Verification items for the finished model (mm, model axes). Face numbers are marked on the shaded views. A direction names the side the tool comes from. Coordinates: 2 decimals unless noted, no trailing zeros. Write each loop counter-clockwise with the first axis right and the second up, starting at its lowest first coordinate (ties: lowest second). Pieces come first, ordered by that corner, then holes. Notation, with made-up numbers: (30.25, -26.75) -> (57.25, -26.75) arc R20 ccw to (57.25, -19.75) -> close; hole circle Ø9 at (88.25, 55.25). An arc over 180 degrees is marked (long way). Answer in a Markdown table with one row per item.
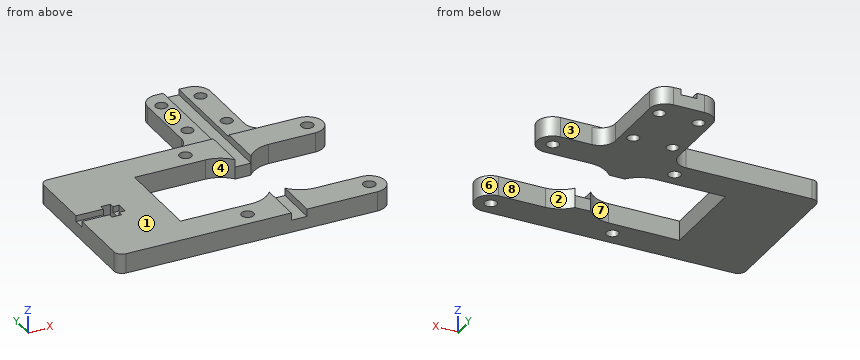
Autodesk Inventor part; units mm, degrees
ref_plane "Arbeitsebene1" through (0, 0, 5) normal (0, 0, 1) x (1, 0, 0)
ref_plane "YZ Plane" through (0, 0, 0) normal (1, 0, 0) x (0, 1, 0)
ref_plane "XZ Plane" through (0, 0, 0) normal (0, 1, 0) x (-1, 0, 0)
sketch "Skizze1" plane through (0, 0, 0) normal (0, 0, 1) x (1, 0, 0)
  line L0 (0, -27.3) -> (0, 27.3)
  line L1 (-71.7, 0) -> (34.7, 0)
  circle A0 centre (-15.5, 15.5) radius 1.55
  circle A1 centre (15.5, 15.5) radius 1.55
  circle A2 centre (-15.5, -15.5) radius 1.55
  circle A3 centre (15.5, -15.5) radius 1.55
  circle A4 centre (-16.5, 0) radius 11
  circle A5 centre (0, 0) radius 5.5
  circle A6 centre (-16.5, 0) radius 4
  arc A7 (-16.5, -7.5) -> (-16.5, 7.5) centre (-16.5, 0) ccw
  line L2 (-16.5, 7.5) -> (-36.5, 7.5)
  line L3 (-36.5, 7.5) -> (-56.5, 7.5)
  line L4 (-56.5, 7.5) -> (-56.5, -7.5)
  line L5 (-56.5, -7.5) -> (-16.5, -7.5)
  circle A8 centre (15.5, 15.5) radius 4
  circle A9 centre (-15.5, 15.5) radius 4
  line L6 (15.5, 11.5) -> (-15.5, 11.5)
  line L7 (15.5, 19.5) -> (-15.5, 19.5)
  line L8 (-15.5, 19.5) -> (-50.5, 19.5)
  line L9 (-15.5, 11.5) -> (-30.5, 11.5)
  line L10 (-50.5, 19.5) -> (-50.5, 0)
  line L11 (-30.5, 11.5) -> (-30.5, 0)
  line L12 (-15.5, -19.5) -> (-50.5, -19.5)
  line L13 (-15.5, -11.5) -> (-30.5, -11.5)
  line L14 (-50.5, -19.5) -> (-50.5, 0)
  line L15 (-30.5, -11.5) -> (-30.5, 0)
  line L16 (15.5, -11.5) -> (-15.5, -11.5)
  line L17 (15.5, -19.5) -> (-15.5, -19.5)
  line L18 (-15.5, -11.5) -> (15.5, -11.5)
  line L19 (15.5, -19.5) -> (-15.5, -19.5)
  line L20 (-30.5, -11.5) -> (15.5, -11.5)
  line L21 (15.5, -19.5) -> (-50.5, -19.5)
  arc A10 (15.5, -19.5) -> (15.5, -11.5) centre (15.5, -15.5) ccw
  point P0 (-50.5, 7.5)
  point P1 (-30.5, 7.5)
  dimension "d0" = 3.1
  dimension "d1" = 15.5
  dimension "d2" = 15.5
  dimension "d3" = 22
  dimension "d4" = 16.5
  dimension "d5" = 11
  dimension "d6" = 8
  dimension "d7" = 15
  dimension "d10" = 15
  dimension "d11" = 40
  dimension "d17" = 8
  dimension "d19" = 8
  dimension "d22" = 35
  dimension "d23" = 15
ref_plane "Arbeitsebene1" through (0, 0, 5) normal (0, 0, 1) x (1, 0, 0)
extrude "Extrusion5" add sketch "Skizze1" along normal blind 5 contours L17 L12 L14 L5 L15 L13 L16 L0 | L0 L16 A10 L17 | L14 L1 L15 L5 | L10 L3 L2 L11 L1 | L6 A9 L7 L0 | L0 L7 A8 L6 | L2 L3 L10 L8 A9 L9 L11 | A8 | A9
sketch "Skizze4" plane through (0, 0, 5) normal (0, 0, 1) x (1, 0, 0)
  line L0 (-30.5, 11.5) -> (15.5, 11.5)
  arc A0 (15.5, 11.5) -> (15.5, 19.5) centre (15.5, 15.5) ccw
  line L1 (15.5, 19.5) -> (-50.5, 19.5)
  line L2 (-50.5, 19.5) -> (-50.5, -19.5)
  line L3 (-50.5, -19.5) -> (15.5, -19.5)
  arc A1 (15.5, -19.5) -> (15.5, -11.5) centre (15.5, -15.5) ccw
  line L4 (15.5, -11.5) -> (-30.5, -11.5)
  line L5 (-30.5, -11.5) -> (-30.5, 11.5)
  circle A2 centre (15.5, 15.5) radius 1.55
  circle A3 centre (15.5, -15.5) radius 1.55
  circle A4 centre (-15.5, -15.5) radius 1.55
  circle A5 centre (-15.5, 15.5) radius 1.55
  line L6 (-64.5, 0) -> (33.5, 0)
  line L7 (-30.5, -11.5) -> (-30.5, 11.5)
  line L8 (-50.5, -1.5) -> (-30.5, -1.5)
  line L9 (-30.5, -1.5) -> (-30.5, 1.5)
  line L10 (-30.5, 1.5) -> (-50.5, 1.5)
  line L11 (-50.5, 1.5) -> (-50.5, -1.5)
  point P0 (0, 0)
  dimension "d34" = 3
extrude "Extrusion8" cut sketch "Skizze4" against normal blind 1.5 contours L5 L6 L2 L10 | L5 L8 L2 L6
sketch "Skizze5" plane through (0, 0, 5) normal (0, 0, 1) x (1, 0, 0)
  line L0 (-50.5, 1.5) -> (-30.5, 1.5)
  line L1 (-30.5, 1.5) -> (-30.5, 11.5)
  line L2 (-30.5, 11.5) -> (15.5, 11.5)
  arc A0 (15.5, 11.5) -> (15.5, 19.5) centre (15.5, 15.5) ccw
  line L3 (15.5, 19.5) -> (-50.5, 19.5)
  line L4 (-50.5, 19.5) -> (-50.5, 1.5)
  circle A1 centre (15.5, 15.5) radius 1.55
  circle A2 centre (-15.5, 15.5) radius 1.55
  circle A3 centre (-15.5, -15.5) radius 1.55
  circle A4 centre (15.5, -15.5) radius 1.55
  line L5 (-30.5, -1.5) -> (-50.5, -1.5)
  line L6 (-50.5, -1.5) -> (-50.5, -19.5)
  line L7 (-50.5, -19.5) -> (15.5, -19.5)
  arc A5 (15.5, -19.5) -> (15.5, -11.5) centre (15.5, -15.5) ccw
  line L8 (15.5, -11.5) -> (-30.5, -11.5)
  line L9 (-30.5, -11.5) -> (-30.5, -1.5)
  line L10 (-30.5, -1.5) -> (-50.5, -1.5)
  line L11 (-30.5, 1.5) -> (-30.5, -1.5)
  line L12 (-50.5, 1.5) -> (-30.5, 1.5)
  line L13 (-50.5, -1.5) -> (-50.5, 1.5)
  line L14 (-64.5, 0) -> (33.5, 0)
  line L15 (-43.5, -2.75) -> (-41.1, -2.75)
  line L16 (-41.1, -2.75) -> (-41.1, 2.75)
  line L17 (-41.1, 2.75) -> (-43.5, 2.75)
  line L18 (-43.5, 2.75) -> (-43.5, -2.75)
  point P0 (0, 0)
  dimension "d37" = 2.4
  dimension "d38" = 5.5
  dimension "d39" = 7
extrude "Extrusion9" cut sketch "Skizze5" against normal blind 3.2 contours L18 L17 L16 L0 | L0 L16 L14 L18 | L14 L16 L5 L18 | L5 L16 L15 L18
sketch "Skizze6" plane through (0, 0, 5) normal (0, 0, 1) x (1, 0, 0)
  line L0 (15.5, 19.5) -> (-50.5, 19.5)
  line L1 (-50.5, -19.5) -> (15.5, -19.5)
  line L2 (-6.4, 19.5) -> (-2.4, 19.5)
  line L3 (-2.4, 19.5) -> (-2.4, -19.5)
  line L4 (-2.4, -19.5) -> (-6.4, -19.5)
  line L5 (-6.4, -19.5) -> (-6.4, 19.5)
  line L6 (-41.1, -1.5) -> (-41.1, -2.75)
  line L7 (-41.1, -2.75) -> (-43.5, -2.75)
  line L8 (-43.5, -2.75) -> (-43.5, -1.5)
  line L9 (-43.5, -1.5) -> (-50.5, -1.5)
  line L10 (-50.5, -1.5) -> (-50.5, -19.5)
  line L11 (-50.5, -19.5) -> (15.5, -19.5)
  arc A0 (15.5, -19.5) -> (15.5, -11.5) centre (15.5, -15.5) ccw
  line L12 (15.5, -11.5) -> (-30.5, -11.5)
  line L13 (-30.5, -11.5) -> (-30.5, -1.5)
  line L14 (-30.5, -1.5) -> (-41.1, -1.5)
  circle A1 centre (15.5, -15.5) radius 1.55
  circle A2 centre (-15.5, -15.5) radius 1.55
  line L15 (0, -27.3) -> (0, 27.3)
  line L16 (-64.5, 0) -> (33.5, 0)
  circle A3 centre (0, 0) radius 3.5191
  dimension "d42" = 4
  dimension "d43" = 2.4
extrude "Extrusion10" cut sketch "Skizze6" against normal blind 1.9 contours L3 A3 L16 L5 L0 | L3 L16 A3 | L16 A3 L3 L12 L5 | L3 A3 L16 | L12 L3 L1 L5
fillet "Rundung1" radius 2 1 edges at (-50.5, -19.5, 2.5)
fillet "Rundung2" radius 2 1 edges at (-50.5, 19.5, 2.5)
sketch "Skizze11" plane through (0, 0, 5) normal (0, 0, 1) x (1, 0, 0)
  line L0 (-2.4, 11.5) -> (-6.4, 11.5)
  line L1 (-2.4, 19.5) -> (-2.4, 11.5)
  line L2 (-6.4, 19.5) -> (-2.4, 19.5)
  line L3 (-6.4, 11.5) -> (-6.4, 19.5)
  arc A0 (-48.5, 19.5) -> (-50.5, 17.5) centre (-48.5, 17.5) ccw
  line L4 (-50.5, 17.5) -> (-50.5, 1.5)
  line L5 (-50.5, 1.5) -> (-43.5, 1.5)
  line L6 (-43.5, 1.5) -> (-43.5, 2.75)
  line L7 (-43.5, 2.75) -> (-41.1, 2.75)
  line L8 (-41.1, 2.75) -> (-41.1, 1.5)
  line L9 (-41.1, 1.5) -> (-30.5, 1.5)
  line L10 (-30.5, 1.5) -> (-30.5, 11.5)
  line L11 (-30.5, 11.5) -> (-6.4, 11.5)
  line L12 (-6.4, 11.5) -> (-6.4, 19.5)
  line L13 (-6.4, 19.5) -> (-48.5, 19.5)
  circle A1 centre (-15.5, 15.5) radius 1.55
  line L14 (-2.4, 19.5) -> (-2.4, 11.5)
  line L15 (-2.4, 11.5) -> (15.5, 11.5)
  arc A2 (15.5, 11.5) -> (15.5, 19.5) centre (15.5, 15.5) ccw
  line L16 (15.5, 19.5) -> (-2.4, 19.5)
  circle A3 centre (15.5, 15.5) radius 1.55
  circle A4 centre (-15.5, -15.5) radius 1.55
  arc A5 (-50.5, -17.5) -> (-48.5, -19.5) centre (-48.5, -17.5) ccw
  line L17 (-48.5, -19.5) -> (-6.4, -19.5)
  line L18 (-6.4, -19.5) -> (-6.4, -11.5)
  line L19 (-6.4, -11.5) -> (-30.5, -11.5)
  line L20 (-30.5, -11.5) -> (-30.5, -1.5)
  line L21 (-30.5, -1.5) -> (-41.1, -1.5)
  line L22 (-41.1, -1.5) -> (-41.1, -2.75)
  line L23 (-41.1, -2.75) -> (-43.5, -2.75)
  line L24 (-43.5, -2.75) -> (-43.5, -1.5)
  line L25 (-43.5, -1.5) -> (-50.5, -1.5)
  line L26 (-50.5, -1.5) -> (-50.5, -17.5)
  line L27 (-6.4, -11.5) -> (-2.4, -11.5)
  line L28 (-6.4, -19.5) -> (-6.4, -11.5)
  line L29 (-2.4, -19.5) -> (-6.4, -19.5)
  line L30 (-2.4, -11.5) -> (-2.4, -19.5)
  line L31 (-2.4, -11.5) -> (-2.4, -19.5)
  line L32 (-2.4, -19.5) -> (15.5, -19.5)
  arc A6 (15.5, -19.5) -> (15.5, -11.5) centre (15.5, -15.5) ccw
  line L33 (15.5, -11.5) -> (-2.4, -11.5)
  circle A7 centre (15.5, -15.5) radius 1.55
  line L34 (-6.4, 11.5) -> (-6.4, 8.5)
  line L35 (-6.4, 8.5) -> (-2.4, 8.5)
  line L36 (-2.4, 8.5) -> (-2.4, 11.5)
  line L37 (-30.5, 11.5) -> (-6.4, 11.5)
  arc A8 (-6.4, 8.5) -> (-12.4, 11.5) centre (-12.6481, 3.5038) ccw
  line L38 (-30.5, 11.5) -> (15.5, 11.5)
  arc A9 (3.6, 11.5) -> (-2.4, 8.5) centre (3.8481, 3.5038) ccw
  line L39 (-64.9971, 0) -> (33.5828, 0)
  line L40 (-6.4, -11.5) -> (-6.4, -8.5)
  line L41 (-6.4, -8.5) -> (-2.4, -8.5)
  line L42 (-2.4, -8.5) -> (-2.4, -11.5)
  arc A10 (-12.4, -11.5) -> (-6.4, -8.5) centre (-12.6481, -3.5038) ccw
  arc A11 (-2.4, -8.5) -> (3.6, -11.5) centre (3.8481, -3.5038) ccw
  circle A12 centre (0, 0) radius 12
  line L43 (-12.4, 11.5) -> (3.6, 11.5)
  line L44 (-12.4, -11.5) -> (3.6, -11.5)
  line L45 (15.5, -11.5) -> (-30.5, -11.5)
  point P0 (0, 0)
  dimension "d61" = 3
  dimension "d62" = 4
  dimension "d63" = 8
  dimension "d64" = 8
  dimension "d65" = 6
  dimension "d66" = 6
extrude "Extrusion13" add sketch "Skizze11" against normal blind 5 contours L36 L35 L34 A12 L0 | L15 A12 A9 L36 | A12 L34 L0 | L15 A9 A12 | L34 A12 A8 L11 | L34 A8 A12 | A12 L33 L42 A11 | A11 L33 A12 | A12 L40 L19 A10 | A10 L40 A12 | L42 L27 A12 L40 L41 | A12 L27 L40
sketch "Skizze12" plane through (0, 0, 5) normal (0, 0, 1) x (1, 0, 0)
  line L0 (-2.4, 11.5) -> (-6.4, 11.5)
  line L1 (-2.4, 19.5) -> (-2.4, 11.5)
  line L2 (-6.4, 19.5) -> (-2.4, 19.5)
  line L3 (-6.4, 11.5) -> (-6.4, 19.5)
  line L4 (-6.4, -11.5) -> (-2.4, -11.5)
  line L5 (-6.4, -19.5) -> (-6.4, -11.5)
  line L6 (-2.4, -19.5) -> (-6.4, -19.5)
  line L7 (-2.4, -11.5) -> (-2.4, -19.5)
  line L8 (-6.4, -11.5) -> (-2.4, -11.5)
  line L9 (-2.4, -11.5) -> (-2.4, 11.5)
  line L10 (-2.4, 11.5) -> (-6.4, 11.5)
  line L11 (-6.4, 11.5) -> (-6.4, -11.5)
  point P0 (0, 0)
extrude "Extrusion14" cut sketch "Skizze12" against normal blind 1.9 contours L9 L4 L11 L0
sketch "Skizze13" plane through (0, 0, 5) normal (0, 0, 1) x (1, 0, 0)
  line L0 (-41.1, 1.5) -> (-41.1, -1.5)
  line L1 (-30.5, -1.5) -> (-41.1, -1.5)
  line L2 (-30.5, 1.5) -> (-30.5, -1.5)
  line L3 (-41.1, 1.5) -> (-30.5, 1.5)
  line L4 (-6.4, -19.5) -> (-6.4, -8.5)
  arc A0 (-12.4, -11.5) -> (-6.4, -8.5) centre (-12.6481, -3.5038) ccw
  line L5 (-12.4, -11.5) -> (-30.5, -11.5)
  line L6 (-30.5, -11.5) -> (-30.5, -1.5)
  line L7 (-30.5, -1.5) -> (-41.1, -1.5)
  line L8 (-41.1, -1.5) -> (-41.1, -2.75)
  line L9 (-41.1, -2.75) -> (-43.5, -2.75)
  line L10 (-43.5, -2.75) -> (-43.5, -1.5)
  line L11 (-43.5, -1.5) -> (-50.5, -1.5)
  line L12 (-50.5, -1.5) -> (-50.5, -17.5)
  arc A1 (-50.5, -17.5) -> (-48.5, -19.5) centre (-48.5, -17.5) ccw
  line L13 (-48.5, -19.5) -> (-6.4, -19.5)
  circle A2 centre (-15.5, -15.5) radius 1.55
  circle A3 centre (-15.5, 15.5) radius 1.55
  line L14 (-6.4, 8.5) -> (-6.4, 19.5)
  line L15 (-6.4, 19.5) -> (-48.5, 19.5)
  arc A4 (-48.5, 19.5) -> (-50.5, 17.5) centre (-48.5, 17.5) ccw
  line L16 (-50.5, 17.5) -> (-50.5, 1.5)
  line L17 (-50.5, 1.5) -> (-43.5, 1.5)
  line L18 (-43.5, 1.5) -> (-43.5, 2.75)
  line L19 (-43.5, 2.75) -> (-41.1, 2.75)
  line L20 (-41.1, 2.75) -> (-41.1, 1.5)
  line L21 (-41.1, 1.5) -> (-30.5, 1.5)
  line L22 (-30.5, 1.5) -> (-30.5, 11.5)
  line L23 (-30.5, 11.5) -> (-12.4, 11.5)
  arc A5 (-6.4, 8.5) -> (-12.4, 11.5) centre (-12.6481, 3.5038) ccw
  line L24 (-41.1, 1.5) -> (-30.5, 1.5)
  line L25 (-30.5, -1.5) -> (-39.5, -1.5)
  line L26 (-39.5, -1.5) -> (-39.5, 1.5)
  line L27 (-39.5, 1.5) -> (-30.5, 1.5)
  line L28 (-30.5, 1.5) -> (-30.5, -1.5)
  point P0 (0, 0)
  dimension "d71" = 9
extrude "Extrusion15" add sketch "Skizze13" against normal blind 1.5 contours L3 L2 L1 L26
sketch "Skizze18" plane through (15.5, 19.5, 5) normal (0, 1, 0) x (1, 0, 0)
  line L0 (-23.9, -5) -> (-15.9, -5)
  line L1 (-17.9, -0.5) -> (-17.9, -1.9)
  line L2 (-17.9, -1.9) -> (-21.9, -1.9)
  line L3 (-21.9, -1.9) -> (-21.9, -0.5)
  line L4 (-17.9, 0) -> (-17.9, 0.5)
  line L5 (-17.9, 1.9) -> (-17.9, 0)
  line L6 (-17.9, 0.5) -> (-11.9, 0.5)
  line L7 (-11.9, 0) -> (-11.9, 5)
  line L8 (-11.9, 0.5) -> (-11.9, 5)
  line L9 (-11.9, 5) -> (-27.9, 5)
  line L10 (-64, 5) -> (0, 5)
  line L11 (-27.9, 5) -> (-27.9, 0.5)
  line L12 (-27.9, 0) -> (-27.9, 5)
  line L13 (-27.9, 0.5) -> (-21.9, 0.5)
  line L14 (-21.9, 0.5) -> (-21.9, 1.9)
  line L15 (-21.9, 1.9) -> (-17.9, 1.9)
  line L16 (-17.9, 1.9) -> (-17.9, 0.5)
  line L17 (-15.9, -0.5) -> (-15.9, -5)
  line L18 (-15.9, -0.5) -> (-17.9, -0.5)
  line L19 (-21.9, -0.5) -> (-23.9, -0.5)
  line L20 (-23.9, -5) -> (-23.9, -0.5)
  point P0 (-15.5, 5)
  dimension "d89" = 0.5
  dimension "d90" = 4.5
extrude "Extrusion18" add sketch "Skizze18" along normal blind 25 contours L15 L14 L13 L11 L9 L7 L6 L5
sketch "Skizze19" plane through (0, 0, 0) normal (0, 0, -1) x (-1, 0, 0)
  circle A0 centre (-0.6, 39.5) radius 1.5
  circle A1 centre (9.4, 39.5) radius 1.5
  circle A2 centre (9.4, 26.5) radius 1.5
  circle A3 centre (-0.6, 26.5) radius 1.5
  point P0 (0, 0)
extrude "Extrusion19" cut sketch "Skizze19" against normal blind 5
fillet "Rundung3" radius 4 4 edges at (3.6, 19.5, 2.25) (3.6, 44.5, 2.25) (-12.4, 44.5, 2.25) (-12.4, 19.5, 2.25)
properties part number "Drückbrücke_U_Gespiegelt" material "ABS-Kunststoff"
1. Section check C-C, the plane y = 30. Record the boundary of the cut face in (x, z).
Geometry says:
| item | result |
|---|---|
| outline | (-12.4, 0) -> (3.6, 0) -> (3.6, 4.5) -> (-2.4, 4.5) -> (-2.4, 3.1) -> (-6.4, 3.1) -> (-6.4, 4.5) -> (-12.4, 4.5) -> close |
2. Section check A-A, the plane y = 39.5. Record the boundary of the cut face in (x, z).
Geometry says:
| item | result |
|---|---|
| outline | (-12.4, 0) -> (-10.9, 0) -> (-10.9, 4.5) -> (-12.4, 4.5) -> close; (-7.9, 0) -> (-0.9, 0) -> (-0.9, 4.5) -> (-2.4, 4.5) -> (-2.4, 3.1) -> (-6.4, 3.1) -> (-6.4, 4.5) -> (-7.9, 4.5) -> close; (2.1, 0) -> (3.6, 0) -> (3.6, 4.5) -> (2.1, 4.5) -> close |
3. Depth check by flat-ended pin: P1, Ø1.5, axis at x = -23, z = 2, coming from the +Y side; P2, Ø1.9, axis at x = -15.5, y = -15.5, coming from the -Z side; P3, Ø5, axis at x = -9.4, y = 39.5, coming from the +Z side; P4, Ø1.2, axis at x = -5, y = -15.5, coming from the +Z side. Enter the tip coordinate at first touch or a pass-through.
Geometry says:
| item | result |
|---|---|
| P1 | y = 19.5 |
| P2 | through |
| P3 | z = 4.5 |
| P4 | z = 3.1 |
4. Mould release check, pull along X, two halves, no side actions. Record for the marked faces 6, 7 and 8: released by +X, released by -X, zero draft, split by the parting line, or undercut.
Geometry says:
| item | result |
|---|---|
| face 6 | released by +X |
| face 7 | undercut |
| face 8 | zero draft |
5. Thickness scan on line 1 (Y direction, x = -4.5, z = 2.1); line 2 (Y direction, x = -30, z = 0.85); line 3 (Y direction, x = -9.4, z = 1.55). Record the ranges inside material, lowest first. Write a range as from..to.
Geometry says:
| item | result |
|---|---|
| line 1 | -19.5..-8.5, 8.5..44.5 |
| line 2 | -19.5..-11.5, 11.5..19.5 |
| line 3 | -19.5..-10.81, 10.81..25, 28..38, 41..44.37 |
6. Section check B-B, the plane x = -18. Record the boundary of the cut face in (y, z).
Geometry says:
| item | result |
|---|---|
| outline | (-19.5, 0) -> (-11.5, 0) -> (-11.5, 5) -> (-19.5, 5) -> close; (11.5, 0) -> (19.5, 0) -> (19.5, 5) -> (11.5, 5) -> close |
7. Tool access check on the marked faces 1, 2, 3, 4 and 5. Record the directions out of +Z, -Z, +X, -X, +Y, -Y that give a thin tool (end or side, any length) a straight path to the whole face; none if there is none.
Geometry says:
| item | result |
|---|---|
| face 1 | +Z, +X, -X, +Y, -Y |
| face 2 | +Z, -Z, +X |
| face 3 | +Z, +X, +Y |
| face 4 | +Z, -Z |
| face 5 | +Z, +X, -X, +Y |
8. Section check D-D, the plane x = -9.4. Record the boundary of the cut face in (y, z), plus the area to 3 significant figures.
Geometry says:
| item | result |
|---|---|
| outline | (-19.5, 0) -> (-10.81, 0) -> (-10.81, 5) -> (-19.5, 5) -> close; (10.81, 0) -> (25, 0) -> (25, 4.5) -> (19.5, 4.5) -> (19.5, 5) -> (10.81, 5) -> close; (28, 0) -> (38, 0) -> (38, 4.5) -> (28, 4.5) -> close; (41, 0) -> (44.37, 0) -> (44.37, 4.5) -> (41, 4.5) -> close |
| area | 172 mm^2 |
